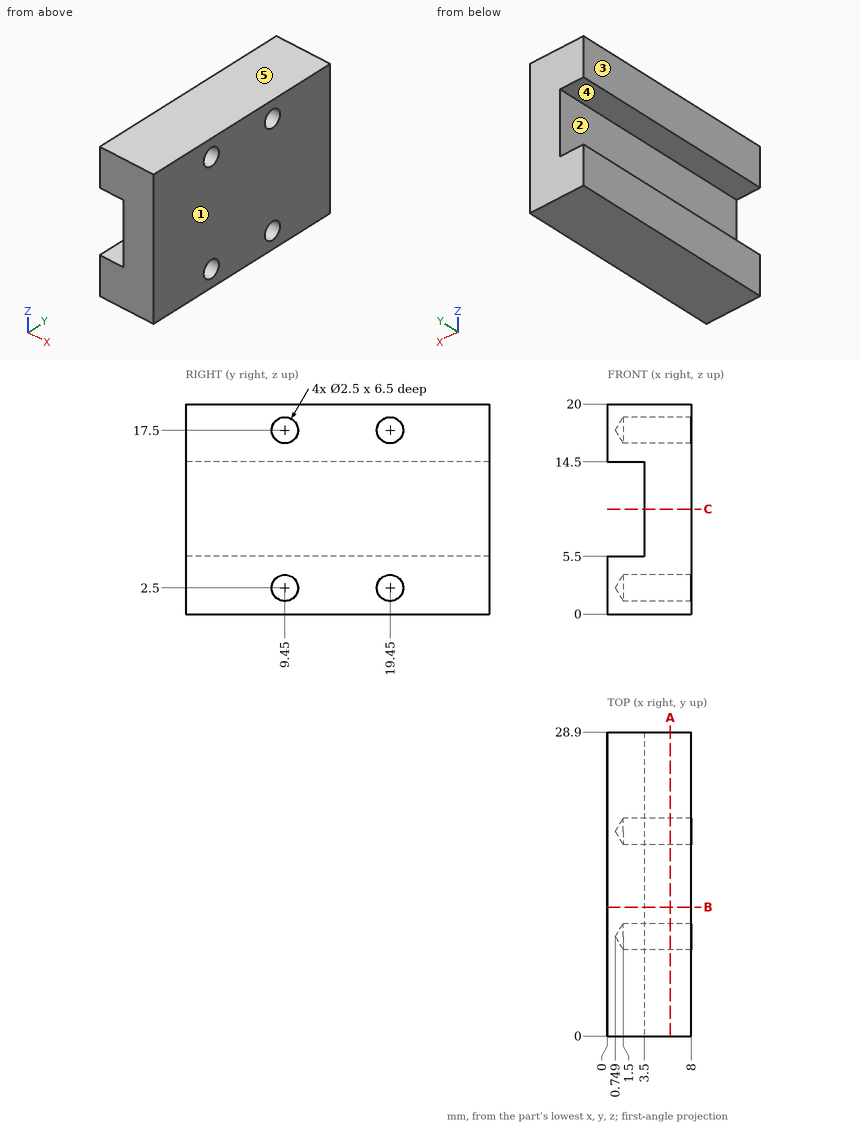
The drawing under review shows one solid part. Ordinate dimensions are in mm from its lowest x, y, z. A direction names the side the tool comes from. Coordinates: 2 decimals unless noted, no trailing zeros. Write each loop counter-clockwise with the first axis right and the second up, starting at its lowest first coordinate (ties: lowest second). Pieces come first, ordered by that corner, then holes. Notation, with made-up numbers: (-38.5, -1.5) -> (-15.5, -1.5) arc R21 cw to (-15.5, 9.5) -> close; hole circle Ø11 at (7, 77). An arc over 180 degrees is marked (long way). Write each question's results on one line, items separated by ' | '. Start each with the question number.
1) Consider section B-B (y = 12.25). Write out the cut boundary in (x, z), plus the area to 4 significant figures.
2) Insertion check: pin 1 (4.5 mm diameter, centred on y = 17.5, z = 10.5, fed in from -X); pin 2 (2 mm diameter, centred on y = 9.45, z = 2.5, fed in from +X). Each pin has a flat end and moves straight along its axis. Give the tip position at first contact, or say it passes through.
3) The part is to be moulded in two halves that separate along Z. For the marked faces 3, 4 and 5, say which applies: +Z half, -Z half, draft (parallel to the pull), parting line (faces both ways), or undercut.
4) Consider section A-A (x = 6). Write out the cut boundary in (y, z).
5) Wall thickness on L1, parallel to Z at x = 6.75, y = 19.45; L2, parallel to Y at x = 3.25, z = 2.5; L3, parallel to Z at x = 3, y = 9.45: over which ranges is each line inside the solid? List them lowest first. Write a range as [from, to].
6) For the marked faces 1 and 2, list the 3-axis set-ups (+Z, -Z, +X, -X, +Y, -Y) from which the entire face can be reached by the end or side of a thin tool; tool diameter is ignored.
7) Consider section C-C (z = 10). Write out the cut boundary in (x, y).
Geometry says:
1) outline: (0, 0) -> (8, 0) -> (8, 20) -> (0, 20) -> (0, 14.5) -> (3.5, 14.5) -> (3.5, 5.5) -> (0, 5.5) -> close | area: 128.5 mm^2
2) pin 1: x = 3.5 | pin 2: x = 1.35
3) face 3: draft | face 4: undercut | face 5: +Z half
4) outline: (0, 0) -> (28.9, 0) -> (28.9, 20) -> (0, 20) -> close; hole circle Ø2.5 at (9.45, 2.5); hole circle Ø2.5 at (9.45, 17.5); hole circle Ø2.5 at (19.45, 2.5); hole circle Ø2.5 at (19.45, 17.5)
5) L1: [0, 1.25], [3.75, 16.25], [18.75, 20] | L2: [0, 8.2], [10.7, 18.2], [20.7, 28.9] | L3: [0, 1.25], [3.75, 5.5], [14.5, 16.25], [18.75, 20]
6) face 1: +Z, -Z, +X, +Y, -Y | face 2: -X, +Y, -Y
7) outline: (3.5, 0) -> (8, 0) -> (8, 28.9) -> (3.5, 28.9) -> close
